```python
from build123d import *
from OCP.BRepFilletAPI import BRepFilletAPI_MakeChamfer

# Parameters (mm, degrees)
SKETCH_1_W      = 145
SKETCH_1_H      = 135
EXTRUDE_1_DEPTH = 5
CHAMFER_1_SIZE  = 5
CHAMFER_1_SIZE2 = 5.553062574
SKETCH_2_W      = 145
SKETCH_2_H      = 98.542875089
EXTRUDE_2_DEPTH = 2
CHAMFER_2_SIZE  = 5
CHAMFER_2_SIZE2 = 5.553062574
SKETCH_3_R      = 5
SKETCH_3_R_2    = 7.5
SKETCH_3_R_3    = 6
EXTRUDE_3_DEPTH = 10
SKETCH_7_R      = 6
SKETCH_7_R_2    = 4
SKETCH_7_R_3    = 8.5
SKETCH_7_R_4    = 6.5
SKETCH_7_R_5    = 7
EXTRUDE_6_DEPTH = 4


with BuildPart() as part:
    # ｽｹｯﾁ1 → 押し出し1 (new body)
    with BuildSketch(Plane(origin=(0, 0, 0), x_dir=(0, 0, -1), z_dir=(1, 0, 0))):
        with Locations((72.5, 67.5)):
            Rectangle(SKETCH_1_W, SKETCH_1_H)
    extrude(amount=EXTRUDE_1_DEPTH)

    # 面取り1: one chamfer whose edges measure the first distance from different faces: ONE call of the kernel's chamfer builder (chamfer() names one face for all edges)
    chamfer_1_edges_1 = [part.edges().sort_by_distance(p)[0] for p in [
        (2.5, 135, 0),
    ]]
    chamfer_1_side_1 = [part.faces().sort_by_distance(p)[0] for p in [
        (2.5, 135, -72.5),
    ]]
    chamfer_1_edges_2 = [part.edges().sort_by_distance(p)[0] for p in [
        (2.5, 135, -145),
    ]]
    chamfer_1_side_2 = [part.faces().sort_by_distance(p)[0] for p in [
        (2.5, 67.5, -145),
    ]]
    chamfer_1_edges_3 = [part.edges().sort_by_distance(p)[0] for p in [
        (2.5, 0, -145),
    ]]
    chamfer_1_side_3 = [part.faces().sort_by_distance(p)[0] for p in [
        (2.5, 0, -72.5),
    ]]
    chamfer_1_edges_4 = [part.edges().sort_by_distance(p)[0] for p in [
        (2.5, 0, 0),
    ]]
    chamfer_1_side_4 = [part.faces().sort_by_distance(p)[0] for p in [
        (2.5, 67.5, 0),
    ]]
    chamfer_1 = BRepFilletAPI_MakeChamfer(part.part.solid().wrapped)
    for e in chamfer_1_edges_1:
        chamfer_1.Add(CHAMFER_1_SIZE, CHAMFER_1_SIZE2, e.wrapped, chamfer_1_side_1[0].wrapped)  # the first distance lies on this face
    for e in chamfer_1_edges_2:
        chamfer_1.Add(CHAMFER_1_SIZE, CHAMFER_1_SIZE2, e.wrapped, chamfer_1_side_2[0].wrapped)  # the first distance lies on this face
    for e in chamfer_1_edges_3:
        chamfer_1.Add(CHAMFER_1_SIZE, CHAMFER_1_SIZE2, e.wrapped, chamfer_1_side_3[0].wrapped)  # the first distance lies on this face
    for e in chamfer_1_edges_4:
        chamfer_1.Add(CHAMFER_1_SIZE, CHAMFER_1_SIZE2, e.wrapped, chamfer_1_side_4[0].wrapped)  # the first distance lies on this face
    add(Compound.cast(chamfer_1.Shape()), mode=Mode.REPLACE)

    # ｽｹｯﾁ2 → 押し出し2 (add)
    with BuildSketch(Plane.ZY):
        with Locations((-72.5, 49.271437545)):
            Rectangle(SKETCH_2_W, SKETCH_2_H)
    extrude(amount=EXTRUDE_2_DEPTH)

    # 面取り2: one chamfer whose edges measure the first distance from different faces: ONE call of the kernel's chamfer builder (chamfer() names one face for all edges)
    chamfer_2_edges_1 = [part.edges().sort_by_distance(p)[0] for p in [
        (-1, 0, -145),
    ]]
    chamfer_2_side_1 = [part.faces().sort_by_distance(p)[0] for p in [
        (1.658082608, 63.325171213, -145),
    ]]
    chamfer_2_edges_2 = [part.edges().sort_by_distance(p)[0] for p in [
        (-1, 0, 0),
    ]]
    chamfer_2_side_2 = [part.faces().sort_by_distance(p)[0] for p in [
        (1.44516378, 0, -72.693189796),
    ]]
    chamfer_2_edges_3 = [part.edges().sort_by_distance(p)[0] for p in [
        (-1, 98.542875089, 0),
    ]]
    chamfer_2_side_3 = [part.faces().sort_by_distance(p)[0] for p in [
        (1.658082608, 62.905146639, 0),
    ]]
    chamfer_2_edges_4 = [part.edges().sort_by_distance(p)[0] for p in [
        (-1, 98.542875089, -145),
    ]]
    chamfer_2_side_4 = [part.faces().sort_by_distance(p)[0] for p in [
        (-1, 98.542875089, -72.5),
    ]]
    chamfer_2 = BRepFilletAPI_MakeChamfer(part.part.solid().wrapped)
    for e in chamfer_2_edges_1:
        chamfer_2.Add(CHAMFER_2_SIZE, CHAMFER_2_SIZE2, e.wrapped, chamfer_2_side_1[0].wrapped)  # the first distance lies on this face
    for e in chamfer_2_edges_2:
        chamfer_2.Add(CHAMFER_2_SIZE, CHAMFER_2_SIZE2, e.wrapped, chamfer_2_side_2[0].wrapped)  # the first distance lies on this face
    for e in chamfer_2_edges_3:
        chamfer_2.Add(CHAMFER_2_SIZE, CHAMFER_2_SIZE2, e.wrapped, chamfer_2_side_3[0].wrapped)  # the first distance lies on this face
    for e in chamfer_2_edges_4:
        chamfer_2.Add(CHAMFER_2_SIZE, CHAMFER_2_SIZE2, e.wrapped, chamfer_2_side_4[0].wrapped)  # the first distance lies on this face
    add(Compound.cast(chamfer_2.Shape()), mode=Mode.REPLACE)

    # ｽｹｯﾁ3 → 押し出し3 (add)
    with BuildSketch(Plane.ZY):
        with Locations((-120.5, 119)):
            Circle(SKETCH_3_R)
        with Locations((-96.5, 119.003353079)):
            Circle(SKETCH_3_R)
        with Locations((-72.5, 119)):
            Circle(SKETCH_3_R)
        with Locations((-48.5, 119)):
            Circle(SKETCH_3_R_2)
        with Locations((-24.5, 119.003353079)):
            Circle(SKETCH_3_R_3)
    extrude(amount=EXTRUDE_3_DEPTH)

    # ｽｹｯﾁ7 → 押し出し6 (add)
    # profile 1 of 5: a face of its own
    with BuildSketch(Plane.ZY.offset(10)):
        with Locations((-120.5, 119)):
            Circle(SKETCH_7_R)
        with Locations((-120.5, 119)):
            Circle(SKETCH_7_R_2, mode=Mode.SUBTRACT)
    # profile 2 of 5: a face of its own
    with BuildSketch(Plane.ZY.offset(10)):
        with Locations((-96.5, 119.003353079)):
            Circle(SKETCH_7_R)
        with Locations((-96.5, 119.003353079)):
            Circle(SKETCH_7_R_2, mode=Mode.SUBTRACT)
    # profile 3 of 5: a face of its own
    with BuildSketch(Plane.ZY.offset(10)):
        with Locations((-72.5, 119)):
            Circle(SKETCH_7_R)
        with Locations((-72.5, 119)):
            Circle(SKETCH_7_R_2, mode=Mode.SUBTRACT)
    # profile 4 of 5: a face of its own
    with BuildSketch(Plane.ZY.offset(10)):
        with Locations((-48.5, 119)):
            Circle(SKETCH_7_R_3)
        with Locations((-48.5, 119)):
            Circle(SKETCH_7_R_4, mode=Mode.SUBTRACT)
    # profile 5 of 5: a face of its own
    with BuildSketch(Plane.ZY.offset(10)):
        with Locations((-24.5, 119.003353079)):
            Circle(SKETCH_7_R_5)
        with Locations((-24.5, 119.003353079)):
            Circle(SKETCH_7_R_2, mode=Mode.SUBTRACT)
    extrude(amount=EXTRUDE_6_DEPTH)


solid = part.part
```
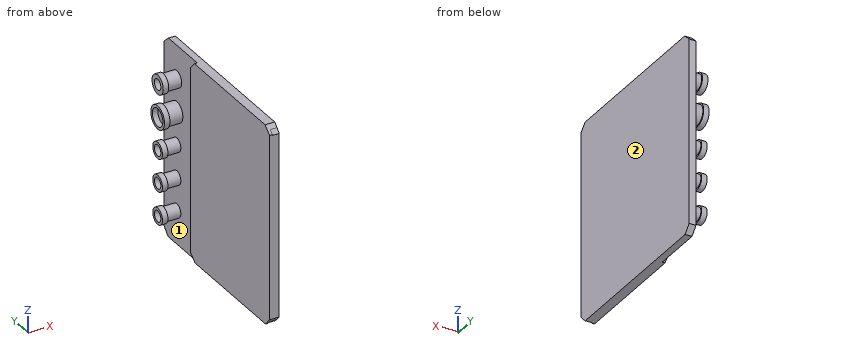
Here's how the part is built. I have some questions about the finished solid (model axes, mm). Face numbers are marked on the shaded views. Coordinates: 2 decimals unless noted, no trailing zeros. Loops run counter-clockwise (first coordinate to the right, second up) from the corner with the lowest first, then second, coordinate; pieces in that order, holes last. Notation, with made-up numbers: (66.5, -22) - (99.5, -22) arc R15 cw to (99.5, 4) - close; hole circle Ø10 at (-28, -19). An arc over 180 degrees is marked (long way). Return JSON: item names as keys, results as strings. Group by question number.
Item 1: If we section it at D-D on z = -96.5: Write out the boundary of the cut face in (x, y), and give its area (3 significant figures).
Item 2: We'd pull the mould along Y, two halves only. Please class the marked faces 1 and 2: +Y half, -Y half, draft (parallel to the pull), parting line (faces both ways), or undercut.
Item 3: If we section it at A-A on z = -24.5: Write out the boundary of the cut face in (x, y), and give its area (3 significant figures).
Item 4: If we section it at B-B on x = -7: Write out the boundary of the cut face in (y, z).
Item 5: Will these pins go through, and if not, where does the flat tip stop? P1, Ø6.5, axis at y = 118, z = -51.5, coming from the -X side; P2, Ø8, axis at x = -7.5, y = 111.5, coming from the +Z side.
Item 6: If we section it at C-C on y = 68: Write out the boundary of the cut face in (x, z).
Item 7: I need wall thicknesses on line 1 (Y direction, x = -11.35, z = -72.5); line 2 (Y direction, x = -12.65, z = -24.5); line 3 (Z direction, x = -6.75, y = 115.5). Which ranges of each line are inside material? Lowest first, please. Write a range as from..to.
Calculated:
{
 "1": {"outline": "(-14, 113) - (-10, 113) - (-10, 114) - (0, 114) - (0, 98.54) - (-2, 98.54) - (-2, 0) - (5, 0) - (5, 135) - (0, 135) - (0, 124) - (-10, 124) - (-10, 125) - (-14, 125) - (-14, 123) - (-10, 123) - (-10, 115) - (-14, 115) - close", "area": "988 mm^2"},
 "2": {"face 1": "undercut", "face 2": "draft"},
 "3": {"outline": "(-14, 112) - (-10, 112) - (-10, 113) - (0, 113) - (0, 98.54) - (-2, 98.54) - (-2, 0) - (5, 0) - (5, 135) - (0, 135) - (0, 125) - (-10, 125) - (-10, 126) - (-14, 126) - (-14, 123) - (-10, 123) - (-10, 115) - (-14, 115) - close", "area": "1,020 mm^2"},
 "4": {"outline": "circle Ø15 at (119, -48.5); circle Ø12 at (119, -24.5); circle Ø10 at (119, -120.5); circle Ø10 at (119, -96.5); circle Ø10 at (119, -72.5)"},
 "5": {"P1": "stops at x = -10", "P2": "stops at z = -19.04"},
 "6": {"outline": "(-2, -145) - (5, -145) - (5, 0) - (-2, 0) - close"},
 "7": {"line 1": "y = 113..115, 123..125", "line 2": "y = 112..115, 123..126", "line 3": "z = -124.07..-116.93, -100.07..-92.93, -76.07..-68.93, -55.13..-41.87, -29.37..-19.63"}
}
